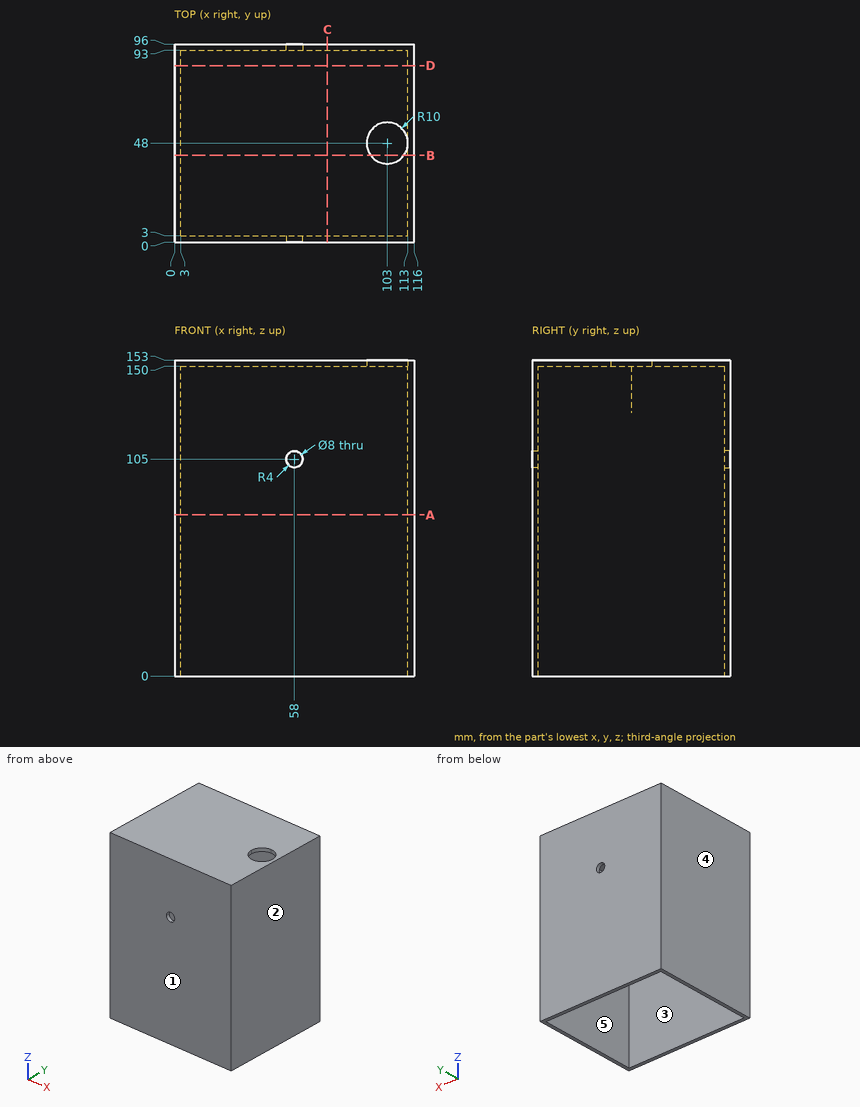
Could you check a few things on this drawing? It's one solid part, dimensions in mm from its lowest x, y, z. A direction names the side the tool comes from. Coordinates: 2 decimals unless noted, no trailing zeros. Loops run counter-clockwise (first coordinate to the right, second up) from the corner with the lowest first, then second, coordinate; pieces in that order, holes last.
1. We'd pull the mould along Y, two halves only. Please class the marked faces 1, 2 and 3: released by +Y, released by -Y, zero draft, split by the parting line, or undercut.
2. Imagine slicing it at D-D (y = 85.5). Please give me the cut outline in (x, z), and give its area (3 significant figures).
3. For P1, Ø8, axis at x = 53, y = 24.5, coming from the -Z side; P2, Ø2, axis at x = 17, z = 137, coming from the -Y side; P3, Ø7, axis at x = 58, z = 105, coming from the +Y side, each with a flat end and sliding along its axis, tell me the tip position at first contact or that it passes through.
4. Imagine slicing it at B-B (y = 42). Please give me the cut outline in (x, z), and give its area (3 significant figures).
5. Imagine slicing it at C-C (x = 74). Please give me the cut outline in (y, z).
6. I need wall thicknesses on L1, parallel to Y at x = 37, z = 127; L2, parallel to X at y = 29.5, z = 74; L3, parallel to X at y = 95.05, z = 105. Which ranges of each line are inside material? Lowest first, please.
7. Imagine slicing it at A-A (z = 78). Please give me the cut outline in (x, y).
8. For the marked faces 4 and 5, which set-ups out of +Z, -Z, +X, -X, +Y, -Y let a thin tool reach every point of the face, with its end or its side?
Computed values:
1. face 1: released by -Y
1. face 2: zero draft
1. face 3: undercut
2. outline: (0, 0) - (3, 0) - (3, 150) - (113, 150) - (113, 0) - (116, 0) - (116, 153) - (0, 153) - close
2. area: 1,250 mm2
3. P1: stops at z = 150
3. P2: stops at y = 0
3. P3: passes through
4. outline: (0, 0) - (3, 0) - (3, 150) - (95, 150) - (95, 153) - (0, 153) - close; (111, 150) - (113, 150) - (113, 0) - (116, 0) - (116, 153) - (111, 153) - close
4. area: 1,200 mm2
5. outline: (0, 0) - (3, 0) - (3, 150) - (93, 150) - (93, 0) - (96, 0) - (96, 153) - (0, 153) - close
6. L1: y = 0 to 3, 93 to 96
6. L2: x = 0 to 3, 113 to 116
6. L3: x = 0 to 54, 62 to 116
7. outline: (0, 0) - (116, 0) - (116, 96) - (0, 96) - close; hole (3, 3) - (113, 3) - (113, 93) - (3, 93) - close
8. face 4: +Z, -Z, -X, +Y, -Y
8. face 5: -Z
